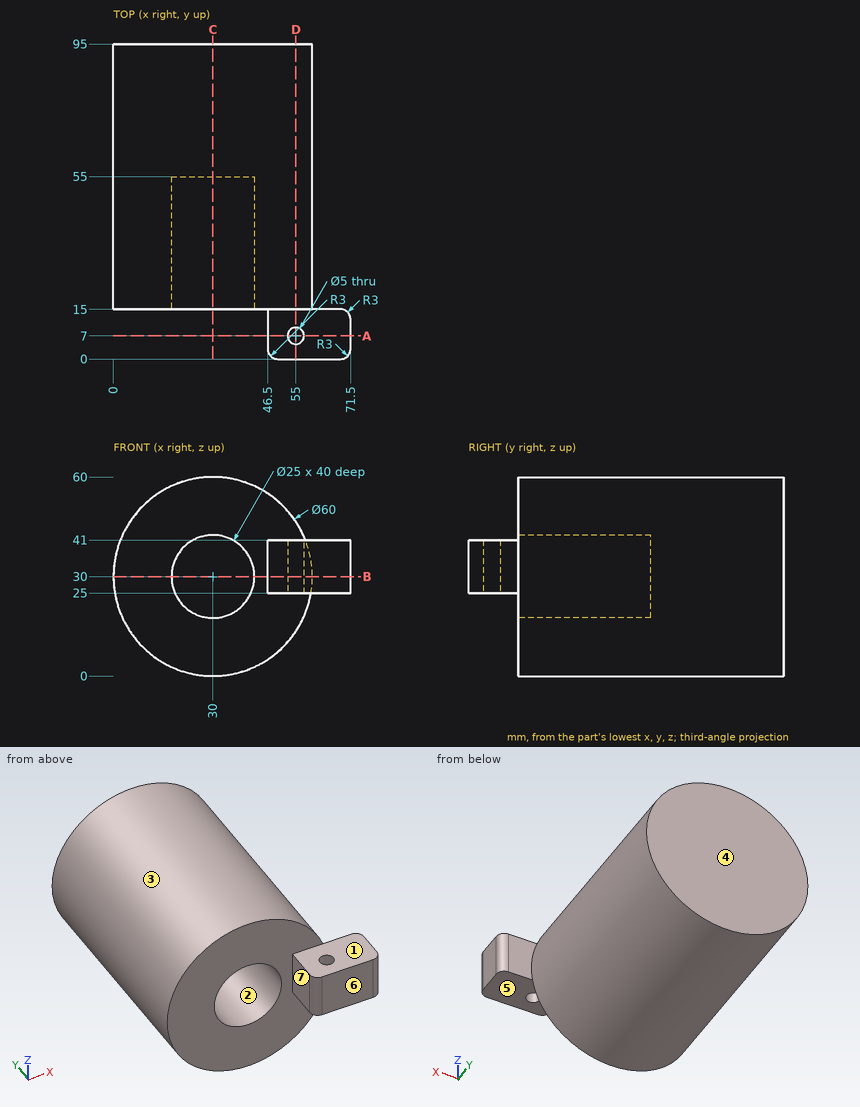
The figure shows three views and two pictorial views of one solid part (mm, origin at its lowest corner). Answer the questions. A direction names the side the tool comes from. Coordinates: 2 decimals unless noted, no trailing zeros. Loops run counter-clockwise (first coordinate to the right, second up) from the corner with the lowest first, then second, coordinate; pieces in that order, holes last.
(1) The part is cut by section C-C (x = 30). Determine the outline of the cut face in (y, z).
Solution:
outline: (15, 0) - (95, 0) - (95, 60) - (15, 60) - (15, 42.5) - (55, 42.5) - (55, 17.5) - (15, 17.5) - close
(2) The part is cut by section D-D (x = 55). Determine the outline of the cut face in (y, z), and give its area (3 significant figures).
Solution:
outline: (0, 25) - (4.5, 25) - (4.5, 41) - (0, 41) - close; (9.5, 25) - (15, 25) - (15, 13.42) - (95, 13.42) - (95, 46.58) - (15, 46.58) - (15, 41) - (9.5, 41) - close
area: 2,810 mm2
(3) Consider line 1 along Z through (x, y) = (30, 44); line 2 along Y through (x, z) = (55, 34.25); line 3 along Y through (x, z) = (18, 18). Determine where each line is inside the solid, lowest interval first.
Solution:
line 1: z = 0 to 17.5, 42.5 to 60
line 2: y = 0 to 4.5, 9.5 to 95
line 3: y = 15 to 95
(4) The mould has two halves that part along Z. Classify the marked faces 1, 2, 3 and 4: released by +Z, released by -Z, zero draft, split by the parting line, or undercut.
Solution:
face 1: released by +Z
face 2: undercut
face 3: split by the parting line
face 4: zero draft
(5) The part is cut by section A-A (y = 7). Determine the outline of the cut face in (x, z).
Solution:
outline: (46.5, 25) - (52.5, 25) - (52.5, 41) - (46.5, 41) - close; (57.5, 25) - (71.5, 25) - (71.5, 41) - (57.5, 41) - close
(6) The part is cut by section B-B (z = 30). Determine the outline of the cut face in (x, y).
Solution:
outline: (0, 15) - (17.5, 15) - (17.5, 55) - (42.5, 55) - (42.5, 15) - (46.5, 15) - (46.5, 3) arc R3 ccw to (49.5, 0) - (68.5, 0) arc R3 ccw to (71.5, 3) - (71.5, 12) arc R3 ccw to (68.5, 15) - (60, 15) - (60, 95) - (0, 95) - close; hole circle Ø5 at (55, 7)
(7) Flat-ended cylindrical pins translate along their axes: pin 1 Ø1 at (x, y) = (17, 26) entering from -Z; pin 2 Ø3 at (x, z) = (64.5, 35) entering from +Y; pin 3 Ø1 at (y, z) = (55.5, 14.5) entering from +X. Find the tip coordinate at first contact, or state that the pin passes through.
Solution:
pin 1: stops at z = 2.73
pin 2: stops at y = 15
pin 3: stops at x = 55.98
(8) A tool of negligible diameter and unlimited length cuts with its end or side. For the marked faces 5, 6 and 7, from which of +Z, -Z, +X, -X, +Y, -Y can it reach the whole face along a straight path? Write none if from no direction.
Solution:
face 5: -Z, +X, -X, -Y
face 6: +Z, -Z, +X, -X, -Y
face 7: +Z, -Z, -X, -Y
